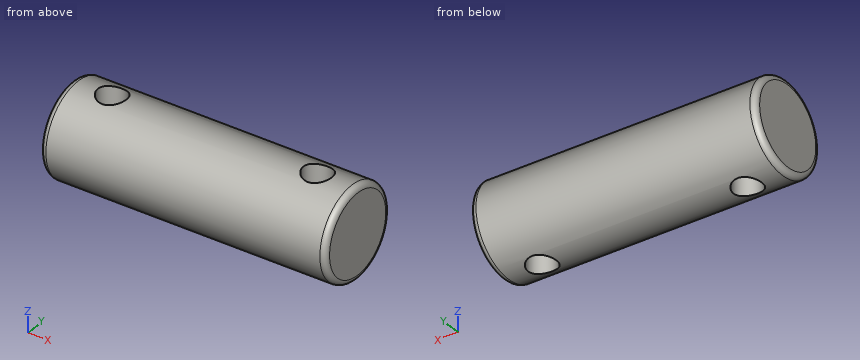
Autodesk Inventor part; units mm, degrees
ref_plane "Work Plane1" through (0, 0, 4.7625) normal (0, 0, 1) x (1, 0, 0)
ref_plane "YZ Plane" through (0, 0, 0) normal (1, 0, 0) x (0, 1, 0)
ref_plane "XZ Plane" through (0, 0, 0) normal (0, 1, 0) x (-1, 0, 0)
sketch "Sketch1" plane through (0, 0, 0) normal (1, 0, 0) x (0, 1, 0)
  circle A0 centre (0, 0) radius 4
  dimension "d0" = 8
extrude "Extrusion1" add sketch "Sketch1" along normal blind 25
fillet "Fillet1" radius 0.5 2 edges at (0, -4, 0) (25, -4, 0)
ref_plane "Work Plane1" through (0, 0, 4.7625) normal (0, 0, 1) x (1, 0, 0)
sketch "Sketch2" plane through (0, 0, 4.7625) normal (0, 0, 1) x (1, 0, 0)
  line L0 (0.5, 4) -> (24.5, 4) construction
  line L1 (12.5, 4) -> (12.5, 0) construction
  line L2 (12.5, 0) -> (21.5, 0) construction
  circle A0 centre (21.5, 0) radius 1.25 construction
  line L3 (12.5, 0) -> (3.5, 0) construction
  circle A1 centre (3.5, 0) radius 1.25 construction
  circle A2 centre (3.5, 0) radius 1.25
  circle A3 centre (21.5, 0) radius 1.25
  point P0 (0, 0)
  dimension "d5" = 9
  dimension "d6" = 2.5
  dimension "d7" = 9
  dimension "d8" = 2.5
  dimension "d9" = 4
extrude "Extrusion2" cut sketch "Sketch2" against normal blind 25
properties part number "Crankshaft Center Rod"
Design review of the part built by this model. Coordinates are the model's own, in mm. Round coordinates to 2 decimals unless told otherwise and drop trailing zeros. Loops run counter-clockwise (first coordinate to the right, second up) from the corner with the lowest first, then second, coordinate; pieces in that order, holes last. Notation, with made-up numbers: (50.25, 21) - (59.25, 21) arc R21 ccw to (59.25, 59) - close; hole circle Ø9 at (-26.5, 83). An arc over 180 degrees is marked (long way). One line per question, with ' | ' between items.
1. For L1, parallel to X at y = 0, z = -1.25; L2, parallel to X at y = -0.75, z = 0.5; L3, parallel to Y at x = 3.5, z = 1, list the stretches that pass through material, from the lowest coordinate up. Write a range as [from, to].
Results are:
L1: x = [0, 2.25], [4.75, 20.25], [22.75, 25] | L2: x = [0, 2.5], [4.5, 20.5], [22.5, 25] | L3: y = [-3.87, -1.25], [1.25, 3.87]
2. We need section A-A, the plane y = 0. State the section outline as (x, z) points, and give its area (3 significant figures).
Results are:
outline: (0, -3.5) arc R0.5 ccw to (0.5, -4) - (2.25, -4) - (2.25, 4) - (0.5, 4) arc R0.5 ccw to (0, 3.5) - close; (4.75, -4) - (20.25, -4) - (20.25, 4) - (4.75, 4) - close; (22.75, -4) - (24.5, -4) arc R0.5 ccw to (25, -3.5) - (25, 3.5) arc R0.5 ccw to (24.5, 4) - (22.75, 4) - close | area: 160 mm²
3. Clearance check with a flat-ended pin moving along its axis: P1, Ø1, axis at x = 6, z = -3, coming from the +Y side. State where the tip first meets the part, or that it passes through.
Results are:
P1: stops at y = 3.12
4. We need section C-C, the plane x = 20.5. State the section outline as (y, z) points, and give its area (3 significant figures).
Results are:
outline: (-0.75, -3.93) - (-0.75, 3.93) arc R4 ccw to start; (0.75, -3.93) arc R4 ccw to (0.75, 3.93) - close | area: 38.3 mm²
5. We need section D-D, the plane x = 6.75. State the section outline as (y, z) points, and give its area (3 significant figures).
Results are:
outline: circle Ø8 at (0, 0) | area: 50.3 mm²
6. We need section B-B, the plane z = 0. State the section outline as (x, y) points, and give its area (3 significant figures).
Results are:
outline: (0, -3.5) arc R0.5 ccw to (0.5, -4) - (24.5, -4) arc R0.5 ccw to (25, -3.5) - (25, 3.5) arc R0.5 ccw to (24.5, 4) - (0.5, 4) arc R0.5 ccw to (0, 3.5) - close; hole circle Ø2.5 at (3.5, 0); hole circle Ø2.5 at (21.5, 0) | area: 190 mm²
